Build history of the part. All positions in model axes, mm. Give positions to 0.01 mm unless a question says otherwise; leave off trailing zeros. Write each loop counter-clockwise with the first axis right and the second up, starting at its lowest first coordinate (ties: lowest second). Pieces come first, ordered by that corner, then holes. Notation, with made-up numbers: (72.25, 73.5) -> (100.25, 73.5) arc R26 cw to (100.25, 101.5) -> close; hole circle Ø5 at (-12, -20). An arc over 180 degrees is marked (long way). Write item = value, one per line. Start each with the question number.
Q1. Saw through at A-A, the plane z = 26.5. List the corners of the cut face in (x, y), then the cut area to 3 significant figures.
Q2. Wall check: line 1 (Z direction, x = -3.5, y = -5.75); line 2 (Z direction, x = 5, y = -12); line 3 (X direction, y = 1.5, z = 28). Give the ranges that are in metal, low to high.
Q3. Drop flat-ended pins along their axis: P1, Ø6, axis at x = -5.5, y = -6, coming from the -Z side; P2, Ø6, axis at x = 4, y = -8.5, coming from the -Z side; P3, Ø1, axis at x = -4, y = 3.5, coming from the -Z side. Give the stop position or say it passes through.
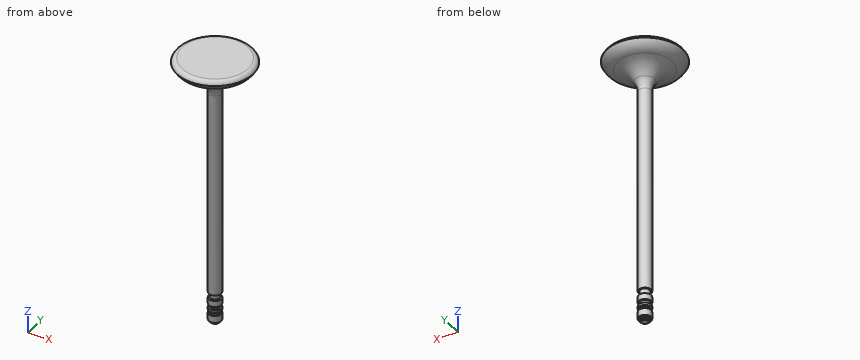
from build123d import *


with BuildPart() as part:
    # Sketch1 → Revolve1 (revolve)
    with BuildSketch(Plane(origin=(0, 0, 0), x_dir=(0, 0, -1), z_dir=(1, 0, 0)), mode=Mode.PRIVATE) as revolve1_sk:
        with BuildLine():
            Line((55.553509337, 0), (-41.692666331, 0))
            Line((-41.692666331, 0), (-41.692666331, 11.814520799))
            ThreePointArc((-41.692666331, 11.814520799), (-41.266642905, 12.931534366), (-40.275497627, 13.6))
            ThreePointArc((-40.275497627, 13.6), (-38.283752535, 11.994111634), (-37.147345345, 9.701841002))
            ThreePointArc((-37.147345345, 9.701841002), (-35.499987602, 6.234951959), (-32.81605757, 3.490935421))
            ThreePointArc((-32.81605757, 3.490935421), (-31.088013134, 2.544687339), (-29.140018683, 2.25))
            Line((-29.140018683, 2.25), (44.382638792, 2.25))
            Line((44.382638792, 2.25), (44.382638792, 1.752462307))
            Line((44.382638792, 1.752462307), (46.11897024, 1.752462307))
            Line((46.11897024, 1.752462307), (46.427430207, 2.25))
            Line((46.427430207, 2.25), (48.58664997, 2.25))
            Line((48.58664997, 2.25), (48.58664997, 1.752462307))
            Line((48.58664997, 1.752462307), (49.573721861, 1.752462307))
            Line((49.573721861, 1.752462307), (49.882181827, 2.25))
            Line((49.882181827, 2.25), (50.745869733, 2.25))
            Line((50.745869733, 2.25), (50.745869733, 2.001231153))
            Line((50.745869733, 2.001231153), (51.147127243, 1.752462307))
            Line((51.147127243, 1.752462307), (51.948863601, 1.752462307))
            Line((51.948863601, 1.752462307), (51.948863601, 2.25))
            Line((51.948863601, 2.25), (54.41654333, 2.25))
            Line((54.41654333, 2.25), (54.41654333, 1.752462307))
            Line((54.41654333, 1.752462307), (55.064309259, 1.752462307))
            Line((55.064309259, 1.752462307), (55.064309259, 1.166388371))
            Line((55.064309259, 1.166388371), (55.553509337, 1.166388371))
            Line((55.553509337, 1.166388371), (55.553509337, 0))
        make_face()
    revolve(revolve1_sk.sketch.rotate(Axis((0, 0, -55.553509337), (0, 0, 1)), 90), axis=Axis((0, 0, -55.553509337), (0, 0, 1)))


solid = part.part
Report:
q1.outline = circle Ø4.5 at (0, 0)
q1.area = 15.9 mm2
q2.line_1 = 35.83 to 41.69
q2.line_2 = 39.31 to 41.21
q2.line_3 = -1.68 to 1.68
q3.P1 = 34.63
q3.P2 = 35.61
q3.P3 = 34.33
